Source: CAD feature listing. Evaluate the final solid. Frame: model axes, mm. A direction names the side the tool comes from. Round coordinates to 2 decimals unless told otherwise and drop trailing zeros. Order: outer loops, then holes, each group sorted by start corner. A loop starts at its lowest first (then second) coordinate and runs counter-clockwise, first axis right, second up. Notation, with made-up numbers: (-20.75, 81.5) -> (12.25, 81.5) arc R19 ccw to (12.25, 112.5) -> close; hole circle Ø11 at (-23, 89). An arc over 180 degrees is marked (long way). One line per item, written item: value. Start each with the question number.
1) Ray query, L1, parallel to Y at x = 0, z = 5.5 (3 decimals); L2, parallel to Z at x = -8.7, y = 0 (3 decimals); L3, parallel to Z at x = 2.5, y = -10.25. Return the intervals inside material, ascending.
2) Section A-A (y = 0). Return the cut outline in (x, z) (3 decimals), and give its area (3 significant figures).
3) Section D-D (z = 15.25). Return the cut outline in (x, y) (3 decimals).
4) Reachability of faces 1 (the face through (9, 4, 6.35)), 2 (the face through (-6, -5, 15.875)) from +Z, -Z, +X, -X, +Y, -Y: full face, straight path, thin tool, end or side. Return the list, or none.
5) Section C-C (y = -7). Return the cut outline in (x, z) (3 decimals), and give its area (3 significant figures).
6) Pin query (flat end, axial travel): P1, Ø1.5, axis at y = 7.5, z = 4.5, coming from the -X side; P2, Ø3, axis at x = -1, z = 2.5, coming from the +Y side (3 decimals); P3, Ø8, axis at x = -7, z = 13, coming from the -Y side; P4, Ø4, axis at x = 3, z = 8.5, coming from the -Y side. Return the tip coordinate at first contact, or that it passes through.
7) Mould query, pull axis Y, two halves, no side actions, for faces 3 (the face through (-9.645, 1.167, 4.448)), 4 (the face through (-6, -5, 0)), 5 (the face through (11.51, 3.62, 3.13)). Classes: pulls with the +Y half, pulls with the -Y half, needs draft (parallel to the pull), parting line crosses it, or undercut.
8) Section B-B (x = -3.25). Return the cut outline in (y, z) (3 decimals).
```python
from build123d import *

# Parameters (mm, degrees)
SKETCH1_R           = 12.065
BOSS_EXTRUDE1_DEPTH = 6.35
SKETCH2_R           = 9.525
BOSS_EXTRUDE2_DEPTH = 9.525
SKETCH3_R           = 7.493
CUT_EXTRUDE1_DEPTH  = 16.875
SKETCH4_R           = 1.7272
CUT_EXTRUDE2_DEPTH  = 13.065


with BuildPart() as part:
    # Sketch1 → Boss-Extrude1 (new body)
    with BuildSketch(Plane.XY):
        Circle(SKETCH1_R)
    extrude(amount=BOSS_EXTRUDE1_DEPTH)

    # Sketch2 → Boss-Extrude2 (add)
    with BuildSketch(Plane.XY.offset(6.35)):
        Circle(SKETCH2_R)
    extrude(amount=BOSS_EXTRUDE2_DEPTH)

    # Sketch3 → Cut-Extrude1 (cut, through all)
    with BuildSketch(Plane(origin=(0, 0, 0), x_dir=(-1, 0, 0), z_dir=(0, 0, -1))):
        Circle(SKETCH3_R)
    extrude(amount=-CUT_EXTRUDE1_DEPTH, mode=Mode.SUBTRACT)

    # Sketch4 → Cut-Extrude2 (cut, through all)
    with BuildSketch(Plane(origin=(0, 0, 0), x_dir=(0, 0, -1), z_dir=(1, 0, 0))):
        with Locations((-3.175, 0)):
            Circle(SKETCH4_R)
    extrude(amount=-CUT_EXTRUDE2_DEPTH, mode=Mode.SUBTRACT)


solid = part.part
```
Findings:
1. L1: -12.065 to -7.493, 7.493 to 12.065
1. L2: 0 to 1.448, 4.902 to 15.875
1. L3: 0 to 6.35
2. outline: (-12.065, 0) -> (-7.493, 0) -> (-7.493, 1.448) -> (-12.065, 1.448) -> close; (-12.065, 4.902) -> (-7.493, 4.902) -> (-7.493, 15.875) -> (-9.525, 15.875) -> (-9.525, 6.35) -> (-12.065, 6.35) -> close; (7.493, 0) -> (12.065, 0) -> (12.065, 6.35) -> (9.525, 6.35) -> (9.525, 15.875) -> (7.493, 15.875) -> close
2. area: 81.0 mm2
3. outline: circle Ø19.05 at (0, 0); hole circle Ø14.986 at (0, 0)
4. face 1: +Z
4. face 2: +Z, +X, -X, +Y, -Y
5. outline: (-9.827, 0) -> (-2.673, 0) -> (-2.673, 15.875) -> (-6.46, 15.875) -> (-6.46, 6.35) -> (-9.827, 6.35) -> close; (2.673, 0) -> (9.827, 0) -> (9.827, 6.35) -> (6.46, 6.35) -> (6.46, 15.875) -> (2.673, 15.875) -> close
5. area: 163 mm2
6. P1: x = -10
6. P2: y = 12.065
6. P3: y = -9.04
6. P4: y = -9.47
7. face 3: undercut
7. face 4: needs draft
7. face 5: parting line crosses it
8. outline: (-11.619, 0) -> (-6.751, 0) -> (-6.751, 15.875) -> (-8.953, 15.875) -> (-8.953, 6.35) -> (-11.619, 6.35) -> close; (6.751, 0) -> (11.619, 0) -> (11.619, 6.35) -> (8.953, 6.35) -> (8.953, 15.875) -> (6.751, 15.875) -> close
